Could you check a few things on this model? Use its own coordinates, in mm. A direction names the side the tool comes from. Coordinates: 2 decimals unless noted, no trailing zeros. Loops run counter-clockwise (first coordinate to the right, second up) from the corner with the lowest first, then second, coordinate; pieces in that order, holes last. Notation, with made-up numbers: (64.25, 49) -> (108.25, 49) arc R28 cw to (108.25, 84) -> close; hole circle Ø8 at (46, 63.5). An arc over 180 degrees is marked (long way). One line per question, with ' | ' between items. Start each with the question number.
(1) Suppose I cut it at B-B (z = 0). Give the number of separate pieces and of enclosed holes in the cut face, plus the area to 3 significant figures.
(2) If we mould it in two halves opening along Z, with no side actions, what happens to faces 1 (the face through (-1, 3, 22.225)), 2 (the face through (35.531, 5.093, 16.757)), 3 (the face through (39.969, 5.093, -14.243)), 4 (the face through (47.625, 3, 0))? For each: pulls with the +Z half, pulls with the -Z half, needs draft (parallel to the pull), parting line crosses it, or undercut.
(3) Suppose I cut it at D-D (x = -19.5). Please give me the cut outline in (y, z) (3 decimals), plus the area to 3 significant figures.
(4) Which directions (+Z, -Z, +X, -X, +Y, -Y) give clear straight access to the entire face, cutting with the end or side of a thin tool? Please do faces 5 (the face through (21.162, 3, 0)), 6 (the face through (-38, 5, -12.95)), 7 (the face through (-22, 6.35, 0)).
(5) I'm going to push flat-ended pins straight in: pin 1 Ø7 at (x, z) = (-30.16, 0) entering from -Y; pin 2 Ø1.6 at (x, z) = (-37.75, -15.5) entering from -Y; pin 3 Ø1.5 at (x, z) = (-36.5, -16) entering from +Y. Where does each tip first touch, or does it pass through?
(6) Suppose I cut it at C-C (x = -7). Please give me the cut outline in (y, z) (3 decimals), plus the area to 3 significant figures.
(7) Suppose I cut it at A-A (x = -37.75). Please give me the cut outline in (y, z) (3 decimals).
(8) If I drill on line 1 along X through (y, z) = (1.9, 15.5) (3 decimals); line 2 along Z through (x, y) = (-37.75, 1.9) (3 decimals); line 3 along Z through (x, y) = (-15, 3.5) (3 decimals), over which ranges is the centre line in solid material (lowest first)?
```python
from build123d import *

# Parameters (mm, degrees)
SKETCH1_R                                         = 1.3
BOSS_EXTRUDE1_DEPTH                               = 6.35
CUT_EXTRUDE1_DEPTH                                = 2.55
CSK_FOR_8_FLAT_HEAD_MACHINE_SCREW_100_D           = 4.4958
CSK_FOR_8_FLAT_HEAD_MACHINE_SCREW_100_CSINK_D     = 8.4328
CSK_FOR_8_FLAT_HEAD_MACHINE_SCREW_100_CSINK_ANGLE = 100
CUT_EXTRUDE2_DEPTH                                = 1
CUT_EXTRUDE2_DEPTH_BACK                           = 7.35


with BuildPart() as part:
    # Sketch1 → Boss-Extrude1 (new body)
    with BuildSketch(Plane(origin=(0, 0, 0), x_dir=(1, 0, 0), z_dir=(0, 1, 0))):
        with BuildLine():
            Line((41.275, 22.225), (-41.275, 22.225))
            ThreePointArc((-41.275, 22.225), (-45.765128061, 20.365128061), (-47.625, 15.875))
            Line((-47.625, 15.875), (-47.625, -15.875))
            ThreePointArc((-47.625, -15.875), (-45.765128061, -20.365128061), (-41.275, -22.225))
            Line((-41.275, -22.225), (41.275, -22.225))
            ThreePointArc((41.275, -22.225), (45.765128061, -20.365128061), (47.625, -15.875))
            Line((47.625, -15.875), (47.625, 15.875))
            ThreePointArc((47.625, 15.875), (45.765128061, 20.365128061), (41.275, 22.225))
        make_face()
        with Locations((-37.75, 15.5)):
            Circle(SKETCH1_R, mode=Mode.SUBTRACT)
        with Locations((37.75, 15.5)):
            Circle(SKETCH1_R, mode=Mode.SUBTRACT)
        with Locations((37.75, -15.5)):
            Circle(SKETCH1_R, mode=Mode.SUBTRACT)
        with Locations((-37.75, -15.5)):
            Circle(SKETCH1_R, mode=Mode.SUBTRACT)
    extrude(amount=BOSS_EXTRUDE1_DEPTH)

    # Sketch2 → Cut-Extrude1 (cut)
    with BuildSketch(Plane(origin=(0, 6.35, 0), x_dir=(1, 0, 0), z_dir=(0, 1, 0))):
        Polygon((-34.805513627, 15.5), (-36.277756814, 18.05), (-39.222243186, 18.05), (-40.694486373, 15.5), (-39.222243186, 12.95), (-36.277756814, 12.95), align=None)
        Polygon((36.277756814, 12.95), (34.805513627, 15.5), (36.277756814, 18.05), (39.222243186, 18.05), (40.694486373, 15.5), (39.222243186, 12.95), align=None)
        Polygon((34.805513627, -15.5), (36.277756814, -18.05), (39.222243186, -18.05), (40.694486373, -15.5), (39.222243186, -12.95), (36.277756814, -12.95), align=None)
        Polygon((-36.277756814, -12.95), (-34.805513627, -15.5), (-36.277756814, -18.05), (-39.222243186, -18.05), (-40.694486373, -15.5), (-39.222243186, -12.95), align=None)
    extrude(amount=-CUT_EXTRUDE1_DEPTH, mode=Mode.SUBTRACT)

    # CSK for #8 Flat Head Machine Screw (100)4 (through all)
    with Locations(Plane(origin=(0, 0, 0), x_dir=(-1, 0, 0), z_dir=(0, -1, 0))):
        with Locations((30.1625, 0), (-30.1625, 0)):
            CounterSinkHole(CSK_FOR_8_FLAT_HEAD_MACHINE_SCREW_100_D / 2, CSK_FOR_8_FLAT_HEAD_MACHINE_SCREW_100_CSINK_D / 2, counter_sink_angle=CSK_FOR_8_FLAT_HEAD_MACHINE_SCREW_100_CSINK_ANGLE)

    # Sketch6 → Cut-Extrude2 (cut, two sides)
    with BuildSketch(Plane.XZ) as cut_extrude2_sk:
        with BuildLine():
            Line((-14.8125, -15.225), (14.8125, -15.225))
            ThreePointArc((14.8125, -15.225), (19.302628061, -13.365128061), (21.1625, -8.875))
            Line((21.1625, -8.875), (21.1625, 8.875))
            ThreePointArc((21.1625, 8.875), (19.302628061, 13.365128061), (14.8125, 15.225))
            Line((14.8125, 15.225), (-14.8125, 15.225))
            ThreePointArc((-14.8125, 15.225), (-19.302628061, 13.365128061), (-21.1625, 8.875))
            Line((-21.1625, 8.875), (-21.1625, -8.875))
            ThreePointArc((-21.1625, -8.875), (-19.302628061, -13.365128061), (-14.8125, -15.225))
        make_face()
    extrude(amount=CUT_EXTRUDE2_DEPTH, mode=Mode.SUBTRACT)
    extrude(cut_extrude2_sk.sketch, amount=-CUT_EXTRUDE2_DEPTH_BACK, mode=Mode.SUBTRACT)


solid = part.part
```
Checks:
1) separate pieces: 4 | enclosed holes: 0 | area: 272 mm^2
2) face 1: pulls with the +Z half | face 2: undercut | face 3: undercut | face 4: needs draft
3) outline: (0, -22.225) -> (6.35, -22.225) -> (6.35, -13.159) -> (0, -13.159) -> close; (0, 13.159) -> (6.35, 13.159) -> (6.35, 22.225) -> (0, 22.225) -> close | area: 115 mm^2
4) face 5: +Y, -Y | face 6: +Y | face 7: +Z, -Z, +X, -X, +Y
5) pin 1: stops at y = 0.6 | pin 2: passes through | pin 3: stops at y = 3.8
6) outline: (0, -22.225) -> (6.35, -22.225) -> (6.35, -15.225) -> (0, -15.225) -> close; (0, 15.225) -> (6.35, 15.225) -> (6.35, 22.225) -> (0, 22.225) -> close | area: 88.9 mm^2
7) outline: (0, -22.225) -> (6.35, -22.225) -> (6.35, -18.05) -> (3.8, -18.05) -> (3.8, -16.8) -> (0, -16.8) -> close; (0, -14.2) -> (3.8, -14.2) -> (3.8, -12.95) -> (6.35, -12.95) -> (6.35, 12.95) -> (3.8, 12.95) -> (3.8, 14.2) -> (0, 14.2) -> close; (0, 16.8) -> (3.8, 16.8) -> (3.8, 18.05) -> (6.35, 18.05) -> (6.35, 22.225) -> (0, 22.225) -> close
8) line 1: x = -47.625 to -39.05, -36.45 to 36.45, 39.05 to 47.625 | line 2: z = -22.225 to -16.8, -14.2 to 14.2, 16.8 to 22.225 | line 3: z = -22.225 to -15.222, 15.222 to 22.225
